Check sheet for the modelled part. Datum: model origin and axes. Units: mm. Round coordinates to 2 decimals unless told otherwise and drop trailing zeros. Order: outer loops, then holes, each group sorted by start corner. A loop starts at its lowest first (then second) coordinate and runs counter-clockwise, first axis right, second up. Notation, with made-up numbers: (88.5, 22) -> (147.5, 22) arc R31 cw to (147.5, 59) -> close; hole circle Ø4 at (-26, 7.5). An arc over 180 degrees is marked (long way). Answer as CSV lines item,"result". Start each with the question number.
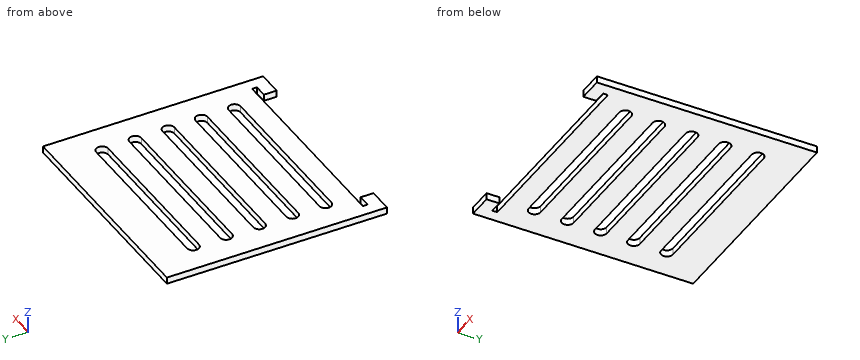
from build123d import *

# Parameters (mm, degrees)
BOSS_EXTRUDE1_DEPTH = 5
LPATTERN1_DEPTH     = 5


# Read off the part's stored shape, not the designer's step: LPattern1
with BuildPart() as part:
    # Sketch1 → Boss-Extrude1 (new body)
    with BuildSketch(Plane.XY):
        Polygon((0, 0), (0, 9.63), (-9.53, 9.63), (-9.53, 13.32), (142.87, 13.32), (142.87, 9.63), (133.34, 9.63), (133.34, 0), (151.95, 0), (151.95, 166.26), (-18.61, 166.26), (-18.61, 0), align=None)
        with BuildLine():
            Line((4.17, 38.509583336), (129.17, 38.509583336))
            ThreePointArc((129.17, 38.509583336), (133.67, 34.009583336), (129.17, 29.509583336))
            Line((129.17, 29.509583336), (4.17, 29.509583336))
            ThreePointArc((4.17, 29.509583336), (-0.33, 34.009583336), (4.17, 38.509583336))
        make_face(mode=Mode.SUBTRACT)
    extrude(amount=BOSS_EXTRUDE1_DEPTH)

    # LPattern1 outline → LPattern1 (cut)
    with BuildSketch(Plane.XY):
        with BuildLine():
            Line((4.17, 129.509583336), (129.17, 129.509583336))
            ThreePointArc((129.17, 129.509583336), (133.67, 134.009583336), (129.17, 138.509583336))
            Line((129.17, 138.509583336), (4.17, 138.509583336))
            ThreePointArc((4.17, 138.509583336), (-0.33, 134.009583336), (4.17, 129.509583336))
        make_face()
        with BuildLine():
            Line((4.17, 104.509583336), (129.17, 104.509583336))
            ThreePointArc((129.17, 104.509583336), (133.67, 109.009583336), (129.17, 113.509583336))
            Line((129.17, 113.509583336), (4.17, 113.509583336))
            ThreePointArc((4.17, 113.509583336), (-0.33, 109.009583336), (4.17, 104.509583336))
        make_face()
        with BuildLine():
            Line((4.17, 79.509583336), (129.17, 79.509583336))
            ThreePointArc((129.17, 79.509583336), (133.67, 84.009583336), (129.17, 88.509583336))
            Line((129.17, 88.509583336), (4.17, 88.509583336))
            ThreePointArc((4.17, 88.509583336), (-0.33, 84.009583336), (4.17, 79.509583336))
        make_face()
        with BuildLine():
            Line((4.17, 54.509583336), (129.17, 54.509583336))
            ThreePointArc((129.17, 54.509583336), (133.67, 59.009583336), (129.17, 63.509583336))
            Line((129.17, 63.509583336), (4.17, 63.509583336))
            ThreePointArc((4.17, 63.509583336), (-0.33, 59.009583336), (4.17, 54.509583336))
        make_face()
    extrude(amount=LPATTERN1_DEPTH, mode=Mode.SUBTRACT)


solid = part.part
1) Section check A-A on x = 18. Record the cut outline in (y, z), then the cut area to 3 significant figures.
2) Section check B-B on z = 2.1. Count the separate pieces of the cut face and the enclosed holes in it, then the cut area to 3 significant figures.
3) Material ranges on line 1 along Y through (x, z) = (123, 3.1); line 2 along Y through (x, z) = (132.5, 1.15); line 3 along Y through (x, z) = (-5, 1.8), recorded low to high.
4) Depth check by flat-ended pin: pin 1 Ø1 at (x, z) = (15, 0.5) entering from -Y; pin 2 Ø12 at (x, y) = (33.5, 87.5) entering from -Z. Enter the tip coordinate at first touch or a pass-through.
Solutions:
1,outline,"(13.32, 0) -> (29.51, 0) -> (29.51, 5) -> (13.32, 5) -> close; (38.51, 0) -> (54.51, 0) -> (54.51, 5) -> (38.51, 5) -> close; (63.51, 0) -> (79.51, 0) -> (79.51, 5) -> (63.51, 5) -> close; (88.51, 0) -> (104.51, 0) -> (104.51, 5) -> (88.51, 5) -> close; (113.51, 0) -> (129.51, 0) -> (129.51, 5) -> (113.51, 5) -> close; (138.51, 0) -> (166.26, 0) -> (166.26, 5) -> (138.51, 5) -> close"
1,area,"540 mm^2"
2,separate pieces,"1"
2,enclosed holes,"5"
2,area,"20,600 mm^2"
3,line 1,"y = 13.32 to 29.51, 38.51 to 54.51, 63.51 to 79.51, 88.51 to 104.51, 113.51 to 129.51, 138.51 to 166.26"
3,line 2,"y = 13.32 to 30.98, 37.04 to 55.98, 62.04 to 80.98, 87.04 to 105.98, 112.04 to 130.98, 137.04 to 166.26"
3,line 3,"y = 0 to 9.63, 13.32 to 166.26"
4,pin 1,"stops at y = 13.32"
4,pin 2,"stops at z = 0"
